The listing builds one solid part. Answer for the finished solid, in the listing's coordinates (mm). Face numbers are marked on the shaded views. A direction names the side the tool comes from. Coordinates: 2 decimals unless noted, no trailing zeros. Order: outer loops, then holes, each group sorted by start corner. A loop starts at its lowest first (then second) coordinate and runs counter-clockwise, first axis right, second up. Notation, with made-up numbers: M -38.75,40 L -28.75,40 A15 ccw -28.75,67 Z; hole C 34,74.5 d6. An arc over 180 degrees is marked long. One line per item, written item: value. Start each with the question number.
Q1. Each of these flat-tipped pins is pushed along its axis until it touches: pin 1 Ø2 at (y, z) = (15, 11.5) entering from +X; pin 2 Ø1 at (x, z) = (6.5, 20) entering from -Y; pin 3 Ø1 at (x, z) = (-22, 3.5) entering from -Y. Where does it stop, or does it pass through?
Q2. For the marked faces 1, 2 and 3, determine the directions among +Z, -Z, +X, -X, +Y, -Y from which every point of the face is accessible in a straight line to the end or side of a thin tool.
Q3. The part is cut by section B-B on y = 33. Give the vertices of the cut face in (x, z), then the cut area to 3 significant figures.
Q4. Straight lines are drawn through the part: line 1 along X through (y, z) = (21.5, 5); line 2 along Y through (x, z) = (7, 7.25); line 3 along Z through (x, y) = (-17.5, 27). For each, find the intervals that lie inside material, in ascending order. Write a range as [from, to].
Q5. The part is cut by section C-C on x = -7. Give the vertices of the cut face in (y, z).
Q6. The part is cut by section D-D on y = 23.5. Give the vertices of the cut face in (x, z), then the cut area to 3 significant figures.
Q7. The part is cut by section A-A on z = 18.25. Give the vertices of the cut face in (x, y) (3 decimals), then the cut area to 3 significant figures.
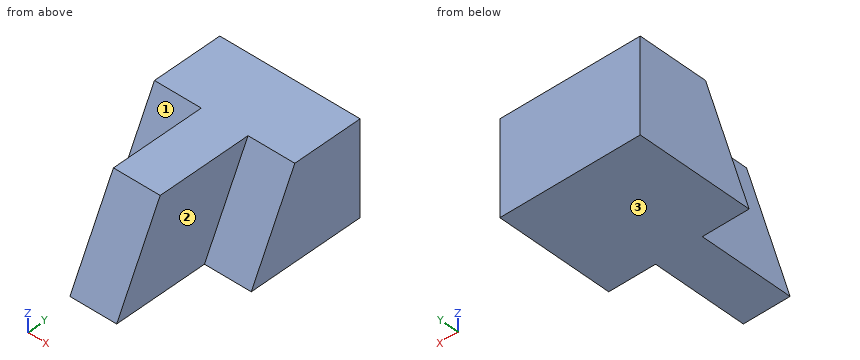
```python
from build123d import *

# Parameters (mm, degrees)
F1_DEPTH = 25.4
F3_DEPTH = 12.7
F5_DEPTH = 12.7
F7_DEPTH = 12.7


with BuildPart() as f1:
    # F0 (on Top) → F1 (new body)
    with BuildSketch(Plane.XY):
        Polygon((10.637409, 57.358576), (0, 57.358576), (-27.462591, 57.358576), (-27.462591, 25.608576), (-14.762591, 25.608576), (-14.762591, 0), (-2.062591, 0), (-2.062591, 25.608576), (10.637409, 25.608576), align=None)
    extrude(amount=F1_DEPTH)

    # F2 (on face) → F3 (cut)
    with BuildSketch(Plane(origin=(-27.462591, 0, 0), x_dir=(0, -1, 0), z_dir=(-1, 0, 0))):
        Polygon((-25.608576, 25.4), (-38.308576, 25.4), (-25.608576, 0), align=None)
    extrude(amount=-F3_DEPTH, mode=Mode.SUBTRACT)

    # F4 (on face) → F5 (cut)
    with BuildSketch(Plane.YZ.offset(10.637409)):
        Polygon((25.608576, 25.4), (25.608576, 0), (38.308576, 25.4), align=None)
    extrude(amount=-F5_DEPTH, mode=Mode.SUBTRACT)

    # F6 (on face) → F7 (cut)
    with BuildSketch(Plane(origin=(-14.762591, 0, 0), x_dir=(0, -1, 0), z_dir=(-1, 0, 0))):
        Polygon((0, 25.4), (-12.7, 25.4), (0, 0), align=None)
    extrude(amount=-F7_DEPTH, mode=Mode.SUBTRACT)


solid = f1.part
```
Output:
1. pin 1: stops at x = -2.06
1. pin 2: stops at y = 35.36
1. pin 3: stops at y = 27.11
2. face 1: +Z, -X, -Y
2. face 2: +Z, +X, -Y
2. face 3: -Z, +X, -X, +Y, -Y
3. outline: M -27.46,0 L 10.64,0 L 10.64,14.78 L -2.06,14.78 L -2.06,25.4 L -14.76,25.4 L -14.76,14.78 L -27.46,14.78 Z
3. area: 698 mm^2
4. line 1: x = [-14.76, -2.06]
4. line 2: y = [29.23, 57.36]
4. line 3: z = [0, 2.78]
5. outline: M 0,0 L 57.36,0 L 57.36,25.4 L 12.7,25.4 Z
6. outline: M -14.76,0 L -2.06,0 L -2.06,25.4 L -14.76,25.4 Z
6. area: 323 mm^2
7. outline: M -27.463,34.734 L -14.763,34.734 L -14.763,9.125 L -2.063,9.125 L -2.063,34.734 L 10.637,34.734 L 10.637,57.359 L -27.463,57.359 Z
7. area: 1,190 mm^2
